Print and shaded views of the part. All mm, measured from the part's lowest x, y and z. A direction names the side the tool comes from. Round coordinates to 2 decimals unless told otherwise and drop trailing zeros. Order: outer loops, then holes, each group sorted by start corner. A loop starts at its lowest first (then second) coordinate and runs counter-clockwise, first axis right, second up. Notation, with made-up numbers: (5, 12.25) - (17, 12.25) arc R26 ccw to (17, 45.25) - close; hole circle Ø3 at (-3.5, -20). An arc over 180 degrees is marked (long way). Write item = value, one per line.
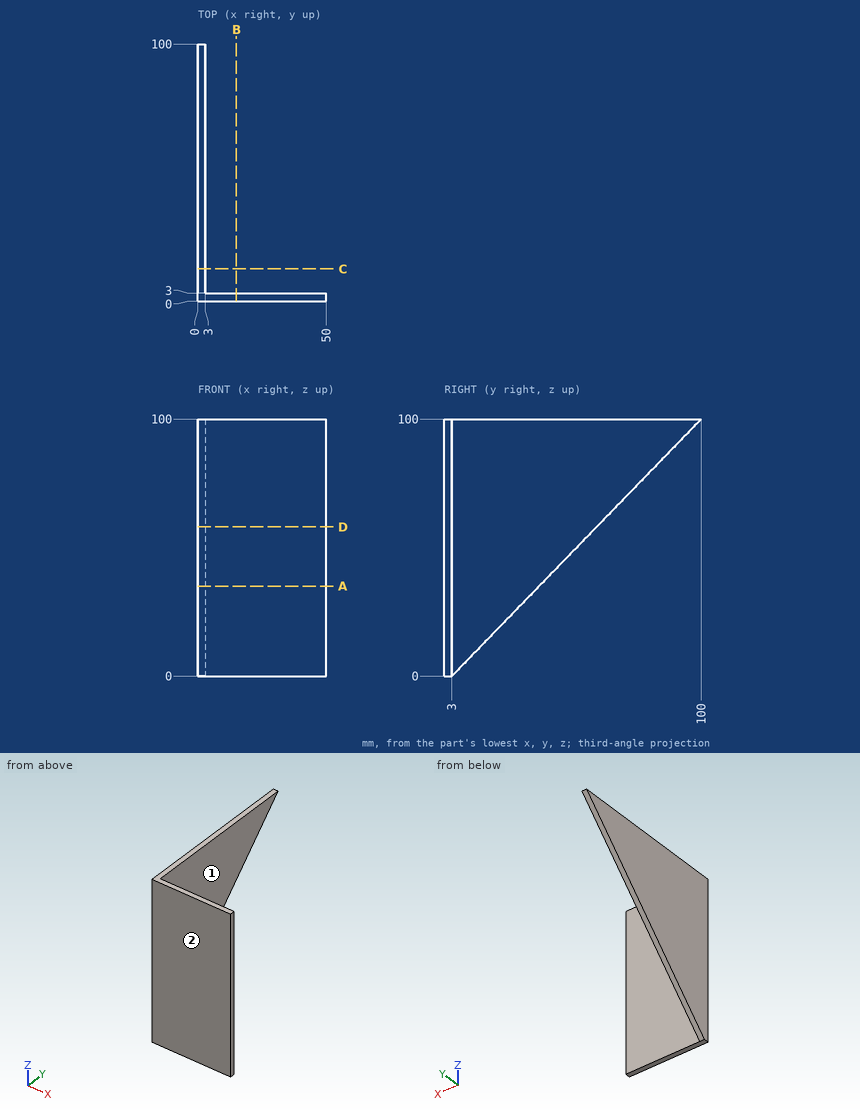
(1) Tool access for the marked faces 1 and 2: list every direction of +Z, -Z, +X, -X, +Y, -Y with a clear straight run to the whole face (end or side of a thin tool).
Solved:
face_1 = +Z, -Z, +X, +Y
face_2 = +Z, -Z, +X, -X, -Y
(2) Band-saw the part on C-C on y = 12.5. List the corners of the cut face in (x, z).
Solved:
outline = (0, 9.79) - (3, 9.79) - (3, 100) - (0, 100) - close
(3) Band-saw the part on B-B on x = 15. List the corners of the cut face in (y, z).
Solved:
outline = (0, 0) - (3, 0) - (3, 100) - (0, 100) - close
(4) Band-saw the part on A-A on z = 35. List the corners of the cut face in (x, y).
Solved:
outline = (0, 0) - (50, 0) - (50, 3) - (3, 3) - (3, 36.95) - (0, 36.95) - close
(5) Drop flat-ended pins along their axis: pin 1 (14 mm diameter, centred on x = 23.5, z = 38.5, fed in from +Y); pin 2 (3 mm diameter, centred on y = 74.5, z = 73, fed in from +X). Give the stop position or say it passes through.
Solved:
pin_1 = 3
pin_2 = 3
(6) Band-saw the part on D-D on z = 58. List the corners of the cut face in (x, y).
Solved:
outline = (0, 0) - (50, 0) - (50, 3) - (3, 3) - (3, 59.26) - (0, 59.26) - close
(7) Probe line 1 along Y through (x, z) = (23, 96.5). List the from-to ranges inside material, lowest first.
Solved:
line_1 = 0 to 3
